from build123d import *
from OCP.BRepFilletAPI import BRepFilletAPI_MakeChamfer

# Parameters (mm, degrees)
SKETCH1_W           = 3.53
SKETCH1_H           = 9.2
BOSS_EXTRUDE1_DEPTH = 4
BOSS_EXTRUDE2_DEPTH = 4
CHAMFER1_SIZE       = 1.5
CHAMFER1_SIZE2      = 0.5


with BuildPart() as part:
    # Sketch1 → Boss-Extrude1 (new body)
    with BuildSketch(Plane.XY):
        Polygon((52.4925, 30), (52.4925, -30), (-54.2075, -30), (-54.2075, 14), (-68.2075, 14), (-68.2075, 30), align=None)
        with BuildLine():
            Line((-31.510630119, 17.647843267), (22.89855475, 17.647843267))
            ThreePointArc((22.89855475, 17.647843267), (-4.306037684, -22.627990687), (-31.510630119, 17.647843267))
        make_face(mode=Mode.SUBTRACT)
        with Locations((-39.0075, 21.35)):
            Rectangle(SKETCH1_W, SKETCH1_H, mode=Mode.SUBTRACT)
        with Locations((45.7925, 20.65)):
            Rectangle(SKETCH1_W, SKETCH1_H, mode=Mode.SUBTRACT)
        with Locations((45.8, -20.65)):
            Rectangle(SKETCH1_W, SKETCH1_H, mode=Mode.SUBTRACT)
        with Locations((-63.9075, 21.35)):
            Rectangle(SKETCH1_W, SKETCH1_H, mode=Mode.SUBTRACT)
    extrude(amount=BOSS_EXTRUDE1_DEPTH)

    # Sketch2 → Boss-Extrude2 (add)
    with BuildSketch(Plane.XY):
        Polygon((-68.2075, 30), (52.4925, 30), (52.4925, 55), (37.4925, 55), (23.350364376, 40.857864376), (-39.065364376, 40.857864376), (-53.2075, 55), (-68.2075, 55), align=None)
    extrude(amount=BOSS_EXTRUDE2_DEPTH)

    # Chamfer1: one chamfer whose edges measure the first distance from different faces: ONE call of the kernel's chamfer builder (chamfer() names one face for all edges)
    chamfer1_edges_1 = [part.edges().sort_by_distance(p)[0] for p in [
        (-40.7725, 21.35, 0),
    ]]
    chamfer1_side_1 = [part.faces().sort_by_distance(p)[0] for p in [
        (-40.7725, 21.35, 2),
    ]]
    chamfer1_edges_2 = [part.edges().sort_by_distance(p)[0] for p in [
        (-39.0075, 16.75, 0),
    ]]
    chamfer1_side_2 = [part.faces().sort_by_distance(p)[0] for p in [
        (-39.0075, 16.75, 2),
    ]]
    chamfer1_edges_3 = [part.edges().sort_by_distance(p)[0] for p in [
        (-37.2425, 21.35, 0),
    ]]
    chamfer1_side_3 = [part.faces().sort_by_distance(p)[0] for p in [
        (-37.2425, 21.35, 2),
    ]]
    chamfer1_edges_4 = [part.edges().sort_by_distance(p)[0] for p in [
        (-39.0075, 25.95, 0),
    ]]
    chamfer1_side_4 = [part.faces().sort_by_distance(p)[0] for p in [
        (-39.0075, 25.95, 2),
    ]]
    chamfer1_edges_5 = [part.edges().sort_by_distance(p)[0] for p in [
        (-65.6725, 21.35, 0),
    ]]
    chamfer1_side_5 = [part.faces().sort_by_distance(p)[0] for p in [
        (-65.6725, 21.35, 2),
    ]]
    chamfer1_edges_6 = [part.edges().sort_by_distance(p)[0] for p in [
        (-63.9075, 16.75, 0),
    ]]
    chamfer1_side_6 = [part.faces().sort_by_distance(p)[0] for p in [
        (-63.9075, 16.75, 2),
    ]]
    chamfer1_edges_7 = [part.edges().sort_by_distance(p)[0] for p in [
        (-62.1425, 21.35, 0),
    ]]
    chamfer1_side_7 = [part.faces().sort_by_distance(p)[0] for p in [
        (-62.1425, 21.35, 2),
    ]]
    chamfer1_edges_8 = [part.edges().sort_by_distance(p)[0] for p in [
        (-63.9075, 25.95, 0),
    ]]
    chamfer1_side_8 = [part.faces().sort_by_distance(p)[0] for p in [
        (-63.9075, 25.95, 2),
    ]]
    chamfer1_edges_9 = [part.edges().sort_by_distance(p)[0] for p in [
        (44.0275, 20.65, 0),
    ]]
    chamfer1_side_9 = [part.faces().sort_by_distance(p)[0] for p in [
        (44.0275, 20.65, 2),
    ]]
    chamfer1_edges_10 = [part.edges().sort_by_distance(p)[0] for p in [
        (45.7925, 16.05, 0),
    ]]
    chamfer1_side_10 = [part.faces().sort_by_distance(p)[0] for p in [
        (45.7925, 16.05, 2),
    ]]
    chamfer1_edges_11 = [part.edges().sort_by_distance(p)[0] for p in [
        (47.5575, 20.65, 0),
    ]]
    chamfer1_side_11 = [part.faces().sort_by_distance(p)[0] for p in [
        (47.5575, 20.65, 2),
    ]]
    chamfer1_edges_12 = [part.edges().sort_by_distance(p)[0] for p in [
        (45.7925, 25.25, 0),
    ]]
    chamfer1_side_12 = [part.faces().sort_by_distance(p)[0] for p in [
        (45.7925, 25.25, 2),
    ]]
    chamfer1_edges_13 = [part.edges().sort_by_distance(p)[0] for p in [
        (47.565, -20.65, 0),
    ]]
    chamfer1_side_13 = [part.faces().sort_by_distance(p)[0] for p in [
        (47.565, -20.65, 2),
    ]]
    chamfer1_edges_14 = [part.edges().sort_by_distance(p)[0] for p in [
        (45.8, -16.05, 0),
    ]]
    chamfer1_side_14 = [part.faces().sort_by_distance(p)[0] for p in [
        (45.8, -16.05, 2),
    ]]
    chamfer1_edges_15 = [part.edges().sort_by_distance(p)[0] for p in [
        (44.035, -20.65, 0),
    ]]
    chamfer1_side_15 = [part.faces().sort_by_distance(p)[0] for p in [
        (44.035, -20.65, 2),
    ]]
    chamfer1_edges_16 = [part.edges().sort_by_distance(p)[0] for p in [
        (45.8, -25.25, 0),
    ]]
    chamfer1_side_16 = [part.faces().sort_by_distance(p)[0] for p in [
        (45.8, -25.25, 2),
    ]]
    chamfer1 = BRepFilletAPI_MakeChamfer(part.part.solid().wrapped)
    for e in chamfer1_edges_1:
        chamfer1.Add(CHAMFER1_SIZE, CHAMFER1_SIZE2, e.wrapped, chamfer1_side_1[0].wrapped)  # the first distance lies on this face
    for e in chamfer1_edges_2:
        chamfer1.Add(CHAMFER1_SIZE, CHAMFER1_SIZE2, e.wrapped, chamfer1_side_2[0].wrapped)  # the first distance lies on this face
    for e in chamfer1_edges_3:
        chamfer1.Add(CHAMFER1_SIZE, CHAMFER1_SIZE2, e.wrapped, chamfer1_side_3[0].wrapped)  # the first distance lies on this face
    for e in chamfer1_edges_4:
        chamfer1.Add(CHAMFER1_SIZE, CHAMFER1_SIZE2, e.wrapped, chamfer1_side_4[0].wrapped)  # the first distance lies on this face
    for e in chamfer1_edges_5:
        chamfer1.Add(CHAMFER1_SIZE, CHAMFER1_SIZE2, e.wrapped, chamfer1_side_5[0].wrapped)  # the first distance lies on this face
    for e in chamfer1_edges_6:
        chamfer1.Add(CHAMFER1_SIZE, CHAMFER1_SIZE2, e.wrapped, chamfer1_side_6[0].wrapped)  # the first distance lies on this face
    for e in chamfer1_edges_7:
        chamfer1.Add(CHAMFER1_SIZE, CHAMFER1_SIZE2, e.wrapped, chamfer1_side_7[0].wrapped)  # the first distance lies on this face
    for e in chamfer1_edges_8:
        chamfer1.Add(CHAMFER1_SIZE, CHAMFER1_SIZE2, e.wrapped, chamfer1_side_8[0].wrapped)  # the first distance lies on this face
    for e in chamfer1_edges_9:
        chamfer1.Add(CHAMFER1_SIZE, CHAMFER1_SIZE2, e.wrapped, chamfer1_side_9[0].wrapped)  # the first distance lies on this face
    for e in chamfer1_edges_10:
        chamfer1.Add(CHAMFER1_SIZE, CHAMFER1_SIZE2, e.wrapped, chamfer1_side_10[0].wrapped)  # the first distance lies on this face
    for e in chamfer1_edges_11:
        chamfer1.Add(CHAMFER1_SIZE, CHAMFER1_SIZE2, e.wrapped, chamfer1_side_11[0].wrapped)  # the first distance lies on this face
    for e in chamfer1_edges_12:
        chamfer1.Add(CHAMFER1_SIZE, CHAMFER1_SIZE2, e.wrapped, chamfer1_side_12[0].wrapped)  # the first distance lies on this face
    for e in chamfer1_edges_13:
        chamfer1.Add(CHAMFER1_SIZE, CHAMFER1_SIZE2, e.wrapped, chamfer1_side_13[0].wrapped)  # the first distance lies on this face
    for e in chamfer1_edges_14:
        chamfer1.Add(CHAMFER1_SIZE, CHAMFER1_SIZE2, e.wrapped, chamfer1_side_14[0].wrapped)  # the first distance lies on this face
    for e in chamfer1_edges_15:
        chamfer1.Add(CHAMFER1_SIZE, CHAMFER1_SIZE2, e.wrapped, chamfer1_side_15[0].wrapped)  # the first distance lies on this face
    for e in chamfer1_edges_16:
        chamfer1.Add(CHAMFER1_SIZE, CHAMFER1_SIZE2, e.wrapped, chamfer1_side_16[0].wrapped)  # the first distance lies on this face
    add(Compound.cast(chamfer1.Shape()), mode=Mode.REPLACE)


solid = part.part
Can you work these out from the model? Positions are in its coordinate system, mm. A direction names the side the tool comes from. Give positions to 0.01 mm unless a question says otherwise; leave off trailing zeros. Write each loop counter-clockwise with the first axis right and the second up, starting at its lowest first coordinate (ties: lowest second). Pieces come first, ordered by that corner, then holes. Notation, with made-up numbers: M -19.5,3.5 L 31.5,3.5 A8 ccw 31.5,11.5 Z; hole C 41,-19 d5. An arc over 180 degrees is marked long. Answer in a Markdown table with one row per item. Add a question column.
Item 1: We'd pull the mould along X, two halves only. Please class faces 4 (the flat face through (-68.208, 35, 2)), 5 (the flat face through (-61, 55, 2)), 6 (the flat face through (-7, 40.858, 2)), 7 (the flat face through (52.492, 12, 2)): released by +X, released by -X, zero draft, split by the parting line, or undercut.
Item 2: Imagine slicing it at A-A, the plane x = 20. Write out the boundary of the cut face in (y, z).
Item 3: Imagine slicing it at D-D, the plane y = 44.5. Write out the boundary of the cut face in (x, z).
Item 4: On a 3-axis mill with a long thin cutter (end or side, diameter ignored), from which of +Z, -Z, +X, -X, +Y, -Y can I reach the whole of each face in a straight line? I mean faces 1 (the flat face through (30.52, 48.03, 1.97)), 2 (the flat face through (-9, 23, 0)), 3 (the flat face through (-65.672, 21, 3)). Say none if no direction works.
Item 5: Imagine slicing it at C-C, the plane y = 22. Write out the boundary of the cut face in (x, z).
Item 6: For pin 1 Ø0.8 at (y, z) = (-21.5, 3) entering from -X; pin 2 Ø0.8 at (x, z) = (-64.5, 2.5) entering from -Y; pin 3 Ø1 at (x, z) = (25, 3.5) entering from +Y, each with a flat end and sliding along its axis, tell me the tip position at first contact or that it passes through.
Item 7: Imagine slicing it at B-B, the plane z = 2.55. State how many separate pieces and enclosed holes the cut face has, plus the area to 3 significant figures.
Item 8: Please list where these lines run through material, in increasing order: L1, parallel to X at y = 24, z = 2.85; L2, parallel to X at y = -20, z = 2.2 (1 decimal); L3, parallel to Y at x = 46.5, z = 1.25.
Evaluation:
| question | item | result |
|---|---|---|
| 1 | face 4 | released by -X |
| 1 | face 5 | zero draft |
| 1 | face 6 | undercut |
| 1 | face 7 | released by +X |
| 2 | outline | M -30,0 L -9.71,0 L -9.71,4 L -30,4 Z; M 17.65,0 L 40.86,0 L 40.86,4 L 17.65,4 Z |
| 3 | outline | M -68.21,0 L -42.71,0 L -42.71,4 L -68.21,4 Z; M 26.99,0 L 52.49,0 L 52.49,4 L 26.99,4 Z |
| 4 | face 1 | +Z, -Z, +Y |
| 4 | face 2 | -Z, +X, -X, +Y, -Y |
| 4 | face 3 | +Z, -Z |
| 5 | outline | M -68.21,0 L -66.17,0 L -65.67,1.5 L -65.67,4 L -68.21,4 Z; M -62.14,1.5 L -61.64,0 L -41.27,0 L -40.77,1.5 L -40.77,4 L -62.14,4 Z; M -37.24,1.5 L -36.74,0 L 43.53,0 L 44.03,1.5 L 44.03,4 L -37.24,4 Z; M 47.56,1.5 L 48.06,0 L 52.49,0 L 52.49,4 L 47.56,4 Z |
| 6 | pin 1 | stops at x = -54.21 |
| 6 | pin 2 | stops at y = 14 |
| 6 | pin 3 | stops at y = 43.01 |
| 7 | separate pieces | 1 |
| 7 | enclosed holes | 5 |
| 7 | area | 6,450 mm² |
| 8 | L1 | x = -68.21 to -65.67, -62.14 to -40.77, -37.24 to 44.03, 47.56 to 52.49 |
| 8 | L2 | x = -54.2 to -16.4, 7.8 to 44, 47.6 to 52.5 |
| 8 | L3 | y = -30 to -25.33, -15.97 to 15.97, 25.33 to 55 |
